Source: CAD feature listing. Evaluate the final solid. Frame: model axes, mm. A direction names the side the tool comes from. Give positions to 0.01 mm unless a question says otherwise; leave off trailing zeros. Write each loop counter-clockwise with the first axis right and the second up, starting at its lowest first coordinate (ties: lowest second). Pieces come first, ordered by that corner, then holes. Notation, with made-up numbers: M 51.25,41 L 62.25,41 A11 ccw 62.25,56 Z; hole C -20.75,67 d6. An arc over 180 degrees is marked long. Return JSON: item names as keys, results as strings.
```python
from build123d import *

# Parameters (mm, degrees)
SKETCH2_R           = 7
BOSS_EXTRUDE1_DEPTH = 2
BOSS_EXTRUDE2_DEPTH = 8
BOSS_EXTRUDE3_DEPTH = 10


with BuildPart() as part:
    # Sketch1 → Revolve1 (revolve)
    with BuildSketch(Plane.XY, mode=Mode.PRIVATE) as revolve1_sk:
        with BuildLine():
            Line((0, 0), (0, 128))
            Line((0, 128), (6, 128))
            Line((6, 128), (6, 20))
            Line((6, 20), (13.597185418, 20))
            ThreePointArc((13.597185418, 20), (20.190643569, 17.518398075), (23.511634032, 11.305261922))
            Line((23.511634032, 11.305261922), (25, 0))
            Line((25, 0), (0, 0))
        make_face()
    revolve(revolve1_sk.sketch.rotate(Axis((0, 0, 0), (0, 1, 0)), 90), axis=Axis((0, 0, 0), (0, 1, 0)))

    # Sketch2 → Boss-Extrude1 (add)
    with BuildSketch(Plane(origin=(0, 0, 0), x_dir=(1, 0, 0), z_dir=(0, 1, 0))):
        with BuildLine():
            Line((-13.516394418, -74.647887324), (-31.377344185, -8.468309859))
            ThreePointArc((-31.377344185, -8.468309859), (0, 32.5), (31.377344185, -8.468309859))
            Line((31.377344185, -8.468309859), (13.516394418, -74.647887324))
            ThreePointArc((13.516394418, -74.647887324), (0, -85), (-13.516394418, -74.647887324))
        make_face()
        with Locations(Location((0, -71, 0), (0, 0, 270))):
            Circle(SKETCH2_R, mode=Mode.SUBTRACT)
    extrude(amount=BOSS_EXTRUDE1_DEPTH)

    # Sketch3 → Boss-Extrude2 (add)
    with BuildSketch(Plane(origin=(0, 20, 0), x_dir=(1, 0, 0), z_dir=(0, 1, 0))):
        Polygon((0, -10.969655115), (9.5, -5.484827557), (9.5, 5.484827557), (0, 10.969655115), (-9.5, 5.484827557), (-9.5, -5.484827557), align=None)
    extrude(amount=BOSS_EXTRUDE2_DEPTH)

    # Sketch5 → Boss-Extrude3 (add)
    with BuildSketch(Plane(origin=(0, 70, 0), x_dir=(1, 0, 0), z_dir=(0, 1, 0))):
        Polygon((0, 10.969655115), (-9.5, 5.484827557), (-9.5, -5.484827557), (0, -10.969655115), (9.5, -5.484827557), (9.5, 5.484827557), align=None)
    extrude(amount=-BOSS_EXTRUDE3_DEPTH)

    # Sketch4 → Cut-Revolve1 (revolve, cut)
    with BuildSketch(Plane(origin=(0, 0, 0), x_dir=(0, 0, -1), z_dir=(1, 0, 0)), mode=Mode.PRIVATE) as cut_revolve1_sk:
        Polygon((8, 20), (10.969655115, 20), (10.969655115, 20.79571669), align=None)
        Polygon((8, 60), (10.969655115, 60), (10.969655115, 60.79571669), align=None)
    revolve(cut_revolve1_sk.sketch.rotate(Axis((0, 60, 0), (0, -1, 0)), 180), axis=Axis((0, 60, 0), (0, -1, 0)), mode=Mode.SUBTRACT)


solid = part.part
```
1) Cut plane D-D, the plane z = 30.5. Return the cut outline in (x, y), then the cut area to 3 significant figures.
Numbers:
{"outline": "M -25.43,0 L 25.43,0 L 25.43,2 L -25.43,2 Z", "area": "102 mm²"}
2) Set-up query: faces 4 (the face through (-2.45, 60.04, 7.77)), 5 (the face through (-9.5, 65, 0)), 6 (the face through (4.684, 65.268, 8.266)), 7 (the face through (9.5, 24, 0)). Return all of +Z, -Z, +X, -X, +Y, -Y with unobstructed straight access to the full face (end or side cutting, diameter ignored); none if empty.
Numbers:
{"face 4": "none", "face 5": "+Z, -Z, -X, +Y", "face 6": "+Z, +X, +Y", "face 7": "+Z, -Z, +X, +Y"}
3) Cut plane B-B, the plane z = 71. Return the cut outline in (x, y), then the cut area to 3 significant figures.
Numbers:
{"outline": "M -14.5,0 L -7,0 L -7,2 L -14.5,2 Z; M 7,0 L 14.5,0 L 14.5,2 L 7,2 Z", "area": "30.0 mm²"}
4) Draft query along Z for faces 1 (the face through (-1.802, 98.594, -5.723)), 2 (the face through (0, 1, 64)), 3 (the face through (-4.684, 24.148, -8.266)). Return one class per face: released by +Z, released by -Z, zero draft, split by the parting line, or undercut.
Numbers:
{"face 1": "split by the parting line", "face 2": "undercut", "face 3": "released by -Z"}
5) Line query: line 1 (Y direction, x = -7.5, z = -5.5); line 2 (Y direction, x = 13, z = 62.5); line 3 (X direction, y = 22.5, z = 5.5). Output: solid intervals per line, ascending. Write a range as [from, to].
Numbers:
{"line 1": "y = [0, 20], [20.35, 28], [60.35, 70]", "line 2": "y = [0, 2]", "line 3": "x = [-9.47, 9.47]"}
6) Cut plane C-C, the plane y = 72. Return the cut outline in (x, z), then the cut area to 3 significant figures.
Numbers:
{"outline": "C 0,0 d12", "area": "113 mm²"}
7) Contact query for flat-ended pins moving along their axis: pin 1 Ø1.5 at (x, z) = (-4, 18.5) entering from +Y; pin 2 Ø5 at (y, z) = (67.5, 2) entering from +X; pin 3 Ø5 at (y, z) = (67.5, 0.5) entering from -X; pin 4 Ø8.5 at (x, z) = (0, 71) entering from +Y. Output: stop coordinate, or through.
Numbers:
{"pin 1": "stops at y = 18.89", "pin 2": "stops at x = 9.5", "pin 3": "stops at x = -9.5", "pin 4": "passes through"}
